Source: CAD feature listing. Evaluate the final solid. Frame: model axes, mm. Face numbers are marked on the shaded views. A direction names the side the tool comes from. Give positions to 0.01 mm unless a question says otherwise; leave off trailing zeros. Write each loop counter-clockwise with the first axis right and the second up, starting at its lowest first coordinate (ties: lowest second). Pieces come first, ordered by that corner, then holes.
```python
from build123d import *

# Parameters (mm, degrees)
F2_R     = 3.344047
F3_DEPTH = 11.1008


with BuildPart() as f1:
    # F0 (on Right) → F1 (revolve)
    with BuildSketch(Plane.YZ):
        Polygon((0.085442, 7.236881), (0, 5.203378), (15.875, 5.203378), (15.875, 8.552678), (14.351, 8.552678), (14.351, 17.763254), (4.7752, 17.763254), (4.7752, 7.236881), align=None)
    revolve(axis=Axis((0, -0.811693, 0), (0, 1, 0)))

    # F2 (on face) → F3 (cut, through all)
    with BuildSketch(Plane.XZ.offset(-4.7752)):
        with Locations((0, 12.318773)):
            Circle(F2_R)
        with Locations((-12.318773, 0)):
            Circle(F2_R)
        with Locations((0, -12.318773)):
            Circle(F2_R)
        with Locations((12.318773, 0)):
            Circle(F2_R)
    extrude(amount=-F3_DEPTH, mode=Mode.SUBTRACT)


solid = f1.part
```
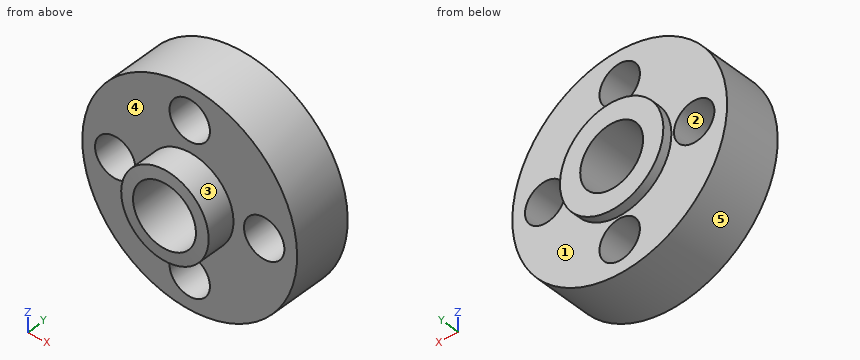
1. Mould query, pull axis X, two halves, no side actions, for the marked faces 1, 2 and 3. Classes: +X half, -X half, draft (parallel to the pull), parting line (faces both ways), or undercut.
2. Cut plane B-B, the plane x = 0. Return the cut outline in (y, z) (3 decimals), then the cut area to 3 significant figures.
3. Cut plane A-A, the plane z = 0. Return the cut outline in (x, y) (3 decimals).
4. Access query for the marked faces 4 and 5. Directions: +Z, -Z, +X, -X, +Y, -Y. A direction counts if a zero-diameter tool reaches every point of the face in a straight line with its end or side. Return the directions, or none.
5. Cut plane C-C, the plane z = -13. Return the cut outline in (x, y).
6. Contact query for flat-ended pins moving along their axis: P1, Ø13.5, axis at x = 0, z = 0, coming from the +Y side (3 decimals); P2, Ø10.5, axis at x = 0, z = 12.32, coming from the -Y side; P3, Ø1, axis at x = 10, z = 8, coming from the +Y side; P4, Ø2, axis at x = 7, y = 4, coming from the +Z side. Output: stop coordinate, or through.
7. Line query: L1, parallel to Z at x = 3, y = 11.25; L2, parallel to X at y = 11.5, z = 0.5; L3, parallel to Y at x = 6.5, z = -10. Output: solid intervals per line, ascending.
8. Cut plane D-D, the plane x = 10. Return the cut outline in (y, z).
Response values:
1. face 1: draft
1. face 2: undercut
1. face 3: parting line
2. outline: (0, -5.203) - (0.085, -7.237) - (4.775, -7.237) - (4.775, -8.975) - (14.351, -8.975) - (14.351, -8.553) - (15.875, -8.553) - (15.875, -5.203) - close; (0, 5.203) - (15.875, 5.203) - (15.875, 8.553) - (14.351, 8.553) - (14.351, 8.975) - (4.775, 8.975) - (4.775, 7.237) - (0.085, 7.237) - close; (4.775, -17.763) - (14.351, -17.763) - (14.351, -15.663) - (4.775, -15.663) - close; (4.775, 15.663) - (14.351, 15.663) - (14.351, 17.763) - (4.775, 17.763) - close
2. area: 142 mm2
3. outline: (-17.763, 4.775) - (-15.663, 4.775) - (-15.663, 14.351) - (-17.763, 14.351) - close; (-8.975, 4.775) - (-7.237, 4.775) - (-7.237, 0.085) - (-5.203, 0) - (-5.203, 15.875) - (-8.553, 15.875) - (-8.553, 14.351) - (-8.975, 14.351) - close; (5.203, 0) - (7.237, 0.085) - (7.237, 4.775) - (8.975, 4.775) - (8.975, 14.351) - (8.553, 14.351) - (8.553, 15.875) - (5.203, 15.875) - close; (15.663, 4.775) - (17.763, 4.775) - (17.763, 14.351) - (15.663, 14.351) - close
4. face 4: -Y
4. face 5: +Y, -Y
5. outline: (-12.11, 4.78) - (-3.27, 4.78) - (-3.27, 14.35) - (-12.11, 14.35) - close; (3.27, 4.78) - (12.11, 4.78) - (12.11, 14.35) - (3.27, 14.35) - close
6. P1: stops at y = 15.875
6. P2: stops at y = 0.08
6. P3: stops at y = 14.35
6. P4: stops at z = 16.58
7. L1: z = -17.51 to -13.8, -10.84 to -4.25, 4.25 to 10.84, 13.8 to 17.51
7. L2: x = -17.76 to -15.63, -9.01 to -5.18, 5.18 to 9.01, 15.63 to 17.76
7. L3: y = 4.78 to 14.35
8. outline: (4.78, -14.68) - (14.35, -14.68) - (14.35, -2.41) - (4.78, -2.41) - close; (4.78, 2.41) - (14.35, 2.41) - (14.35, 14.68) - (4.78, 14.68) - close
